Verification items for the finished model (mm, model axes). A direction names the side the tool comes from. Coordinates: 2 decimals unless noted, no trailing zeros. Order: outer loops, then holes, each group sorted by start corner. A loop starts at its lowest first (then second) coordinate and runs counter-clockwise, first axis right, second up. Notation, with made-up numbers: M 21.25,33 L 69.25,33 A21 cw 69.25,47 Z; hole C 53.5,-17.75 d6. An arc over 180 degrees is marked long. Answer as a JSON object with one key per item and string values. Group by question number.
(1) Cross-section at C-C (z = -6). Enter the section's corners in (x, y), plus the area to 3 significant figures.
(2) Gauge pin test, flat ends, axial feed: pin 1 Ø8.5 at (x, z) = (-194, 7.5) entering from +Y; pin 2 Ø2.5 at (x, z) = (-192.5, 9.5) entering from -Y; pin 3 Ø12 at (y, z) = (51, 2.5) entering from -X. Record the tip position at first contact, or that the pin passes through.
(3) Access from +Z, -Z, +X, -X, +Y, -Y to the whole of each face (thin tool, end or side, straight path). Record for faces 1 (the face through (-193, 82.16, 9)), 2 (the face through (-189.12, -91, 9)), 3 (the face through (-187, -84, 5.08)), 4 (the face through (-189.12, 95, 9)), 5 (the face through (-2, 8, 6.35)).
(4) Mould release check, pull along Y, two halves, no side actions. Record for faces 6 (the face through (-193, -73.821, 9)), 7 (the face through (184.15, -1, 0)), 8 (the face through (0, -101.6, 0)): released by +Y, released by -Y, zero draft, split by the parting line, or undercut.
(5) Cross-section at A-A (x = 132.5). Enter the section's corners in (y, z), plus the area to 3 significant figures.
(6) Material ranges on line 1 (X direction, y = 43, z = 8); line 2 (Y direction, x = 89, z = 11.75); line 3 (X direction, y = 21.5, z = 3.75), recorded low to high.
(7) Cross-section at B-B (y = 55.5). Enter the section's corners in (x, z), plus the area to 3 significant figures.
from build123d import *

# Parameters (mm, degrees)
SKETCH1_W           = 368.3
SKETCH1_H           = 203.2
BOSS_EXTRUDE1_DEPTH = 12.7
SKETCH2_W           = 317.5
SKETCH2_H           = 165.1
CUT_EXTRUDE1_DEPTH  = 6.35
BOSS_EXTRUDE3_DEPTH = 7.62
CUT_EXTRUDE2_DEPTH  = 20.32


with BuildPart() as part:
    # Sketch1 → Boss-Extrude1 (new, symmetric)
    with BuildSketch(Plane.XY):
        Rectangle(SKETCH1_W, SKETCH1_H)
    extrude(amount=BOSS_EXTRUDE1_DEPTH, both=True)

    # Sketch2 → Cut-Extrude1 (cut)
    with BuildSketch(Plane.XY.offset(12.7)):
        with Locations((0, 6.35)):
            Rectangle(SKETCH2_W, SKETCH2_H)
    extrude(amount=-CUT_EXTRUDE1_DEPTH, mode=Mode.SUBTRACT)

    # Sketch4 → Boss-Extrude3 (add)
    with BuildSketch(Plane.XY.offset(12.7)):
        Polygon((184.15, -101.6), (189.119700693, -101.6), (189.119700693, -80.560215749), (197.392455233, -80.560215749), (197.392455233, -89.3698935), (202.362155926, -89.3698935), (202.362155926, -73.820655617), (184.15, -73.820655617), align=None)
        Polygon((189.119700693, 88.9), (197.392455233, 88.9), (197.392455233, 97.709677751), (202.362155926, 97.709677751), (202.362155926, 82.160439868), (184.15, 82.160439868), (184.15, 88.012590692), (184.15, 101.584884773), (189.119700693, 101.584884773), align=None)
    boss_extrude3 = extrude(amount=-BOSS_EXTRUDE3_DEPTH)

    # Mirror2: Boss-Extrude3 across plane
    add(boss_extrude3.mirror(Plane(origin=(0, 0, 0), x_dir=(0, 0, 1), z_dir=(1, 0, 0))))

    # Sketch5 → Cut-Extrude2 (cut)
    with BuildSketch(Plane.XY.offset(12.7)):
        Polygon((202.362155926, -73.820655617), (184.15, -73.820655617), (184.15, -101.6), (189.119700693, -101.6), (189.119700693, -80.560215749), (197.392455233, -80.560215749), (197.392455233, -89.3698935), (202.362155926, -89.3698935), align=None)
        Polygon((184.15, 101.584884773), (184.15, 82.160439868), (202.362155926, 82.160439868), (202.362155926, 97.709677751), (197.392455233, 97.709677751), (197.392455233, 88.9), (189.119700693, 88.9), (189.119700693, 101.584884773), align=None)
    extrude(amount=-CUT_EXTRUDE2_DEPTH, mode=Mode.SUBTRACT)


solid = part.part
Taken from the geometry:
{
 "1": {"outline": "M -184.15,-101.6 L 184.15,-101.6 L 184.15,101.6 L -184.15,101.6 Z", "area": "74,800 mm²"},
 "2": {"pin 1": "stops at y = 97.71", "pin 2": "stops at y = -80.56", "pin 3": "stops at x = -184.15"},
 "3": {"face 1": "+Z, -Z, -X", "face 2": "+Z, -Z, -Y", "face 3": "-Z, -X, +Y, -Y", "face 4": "+Z, -Z, +Y", "face 5": "+Z"},
 "4": {"face 6": "undercut", "face 7": "zero draft", "face 8": "released by -Y"},
 "5": {"outline": "M -101.6,-12.7 L 101.6,-12.7 L 101.6,12.7 L 88.9,12.7 L 88.9,6.35 L -76.2,6.35 L -76.2,12.7 L -101.6,12.7 Z", "area": "4,110 mm²"},
 "6": {"line 1": "x = -184.15 to -158.75, 158.75 to 184.15", "line 2": "y = -101.6 to -76.2, 88.9 to 101.6", "line 3": "x = -184.15 to 184.15"},
 "7": {"outline": "M -184.15,-12.7 L 184.15,-12.7 L 184.15,12.7 L 158.75,12.7 L 158.75,6.35 L -158.75,6.35 L -158.75,12.7 L -184.15,12.7 Z", "area": "7,340 mm²"}
}
